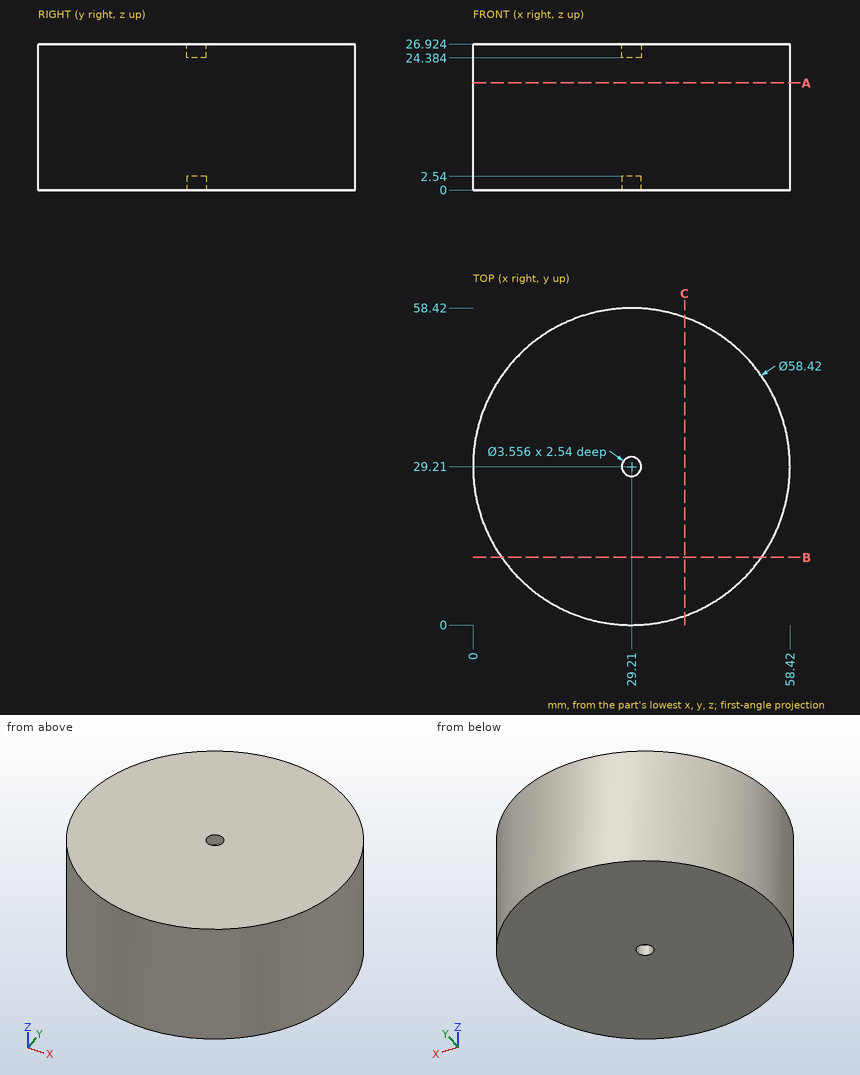
Geometry check sheet. Reference: drawing and pictorial views, mm from the part's lowest x, y, z. Give positions to 0.01 mm unless a question says otherwise; leave off trailing zeros. Loops run counter-clockwise (first coordinate to the right, second up) from the corner with the lowest first, then second, coordinate; pieces in that order, holes last. Notation, with made-up numbers: (-5, 83.25) - (47, 83.25) arc R23 cw to (47, 115.25) - close; hole circle Ø6 at (-16.5, -34). An arc over 180 degrees is marked (long way). One line per question, with ' | ' between items. Start each with the question number.
1. Cross-section at C-C, the plane x = 39. Enter the section's corners in (y, z), plus the area to 3 significant figures.
2. Cross-section at B-B, the plane y = 12.5. Enter the section's corners in (x, z).
3. Gauge pin test, flat ends, axial feed: pin 1 Ø8 at (x, z) = (26.5, 9) entering from +Y; pin 2 Ø3 at (y, z) = (26.5, 9) entering from -X; pin 3 Ø3 at (x, y) = (29.21, 29.21) entering from +Z. Record the tip position at first contact, or that the pin passes through.
4. Material ranges on line 1 along Y through (x, z) = (29.21, 25.2); line 2 along Y through (x, z) = (30, 15), recorded low to high. Write a range as [from, to].
5. Cross-section at A-A, the plane z = 19.75. Enter the section's corners in (x, y), plus the area to 3 significant figures.
Check result:
1) outline: (1.69, 0) - (56.73, 0) - (56.73, 26.92) - (1.69, 26.92) - close | area: 1,480 mm2
2) outline: (5.25, 0) - (53.17, 0) - (53.17, 26.92) - (5.25, 26.92) - close
3) pin 1: stops at y = 58.42 | pin 2: stops at x = 0.03 | pin 3: stops at z = 24.38
4) line 1: y = [0, 27.43], [30.99, 58.42] | line 2: y = [0.01, 58.41]
5) outline: circle Ø58.42 at (29.21, 29.21) | area: 2,680 mm2
